Could you check a few things on this drawing? It's one solid part, dimensions in mm from its lowest x, y, z. Give positions to 0.01 mm unless a question says otherwise; leave off trailing zeros. Order: outer loops, then holes, each group sorted by start corner. A loop starts at its lowest first (then second) coordinate and runs counter-clockwise, first axis right, second up. Notation, with made-up numbers: (57, -13) -> (72, -13) arc R21 ccw to (72, -1) -> close; hole circle Ø10 at (-32.75, 48). An arc over 180 degrees is marked (long way). Answer as a JSON object with one key per item and string values.
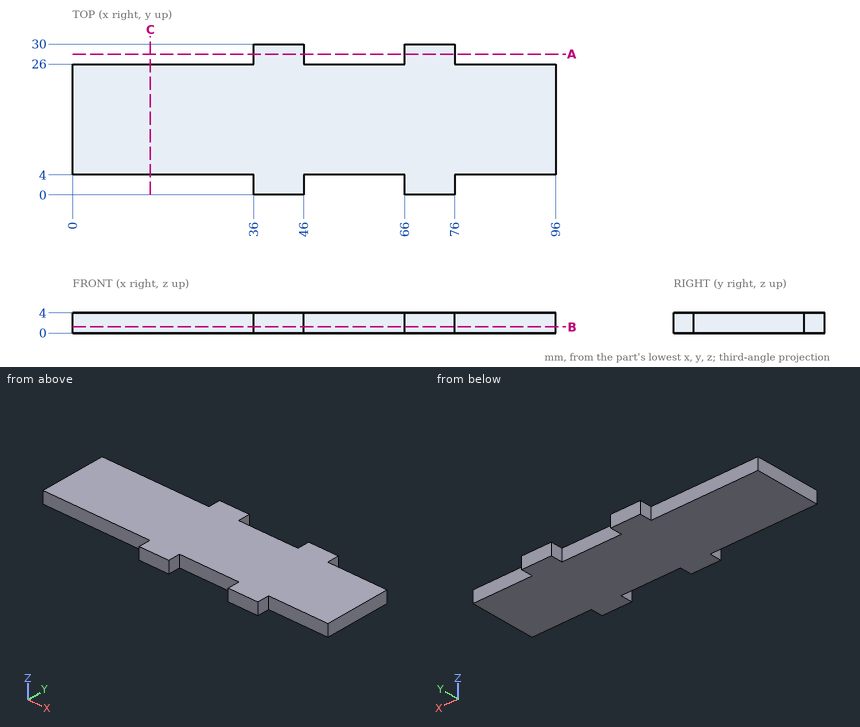
1. If we section it at C-C on x = 15.5: Please give me the cut outline in (y, z), then the cut area to 3 significant figures.
Worked answers:
{"outline": "(4, 0) -> (26, 0) -> (26, 4) -> (4, 4) -> close", "area": "88.0 mm²"}
2. Will these pins go through, and if not, where does the flat tip stop? pin 1 Ø2 at (x, z) = (58, 3) entering from -Y; pin 2 Ø2 at (y, z) = (28.5, 2) entering from -X; pin 3 Ø2 at (y, z) = (28.5, 2.5) entering from +X.
Worked answers:
{"pin 1": "y = 4", "pin 2": "x = 36", "pin 3": "x = 76"}
3. If we section it at A-A on y = 28: Please give me the cut outline in (x, z).
Worked answers:
{"outline": "(36, 0) -> (46, 0) -> (46, 4) -> (36, 4) -> close; (66, 0) -> (76, 0) -> (76, 4) -> (66, 4) -> close"}
4. Please list where this line runs through material, in increasing order: L1, parallel to Y at x = 78, z = 2.05.
Worked answers:
{"L1": "4 to 26"}
5. If we section it at B-B on z = 1.25: Please give me the cut outline in (x, y), then the cut area to 3 significant figures.
Worked answers:
{"outline": "(0, 4) -> (36, 4) -> (36, 0) -> (46, 0) -> (46, 4) -> (66, 4) -> (66, 0) -> (76, 0) -> (76, 4) -> (96, 4) -> (96, 26) -> (76, 26) -> (76, 30) -> (66, 30) -> (66, 26) -> (46, 26) -> (46, 30) -> (36, 30) -> (36, 26) -> (0, 26) -> close", "area": "2,270 mm²"}
